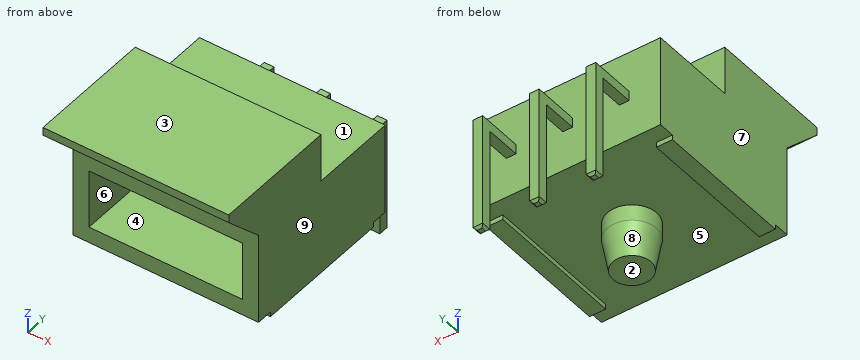
from build123d import *

# Parameters (mm, degrees)
F0_W           = 11.5
F0_H           = 10.66
F0_R           = 1.525
F1_DEPTH       = 5.65
F2_DEPTH       = 3
F3_SIZE2       = 0.3526539614
F3_SIZE        = 2
F4_W           = 9.5
F4_H           = 3.65
F5_DEPTH       = 7
F7_W           = 4.5
F7_H           = 0.6
F7_W_2         = 0.6
F7_H_2         = 4
F7_H_3         = 2.525
F7_W_3         = 5.86
F8_DEPTH       = 0.3
F8_DEPTH_BACK  = 0.3
F10_W          = 10.36
F10_H          = 0.6
F10_W_2        = 0.6
F10_H_2        = 6.525
F11_DEPTH      = 0.3
F11_DEPTH_BACK = 0.3
F13_W          = 10.36
F13_H          = 0.6
F13_W_2        = 0.6
F13_H_2        = 6.525
F14_DEPTH      = 0.3
F14_DEPTH_BACK = 0.3
F15_SIZE       = 0.15
F16_W          = 1
F16_H          = 8.66
F17_DEPTH      = 0.3
F19_DEPTH      = 11.5


with BuildPart() as f1:
    # F0 (on Top) → F1 (new body)
    with BuildSketch(Plane.XY):
        with Locations((0, -2.5)):
            Rectangle(F0_W, F0_H)
        with Locations((0, -2.58)):
            Circle(F0_R, mode=Mode.SUBTRACT)
        with Locations((0, -2.58)):
            Circle(F0_R)
    extrude(amount=F1_DEPTH)

    # F0 (on Top) → F2 (join)
    with BuildSketch(Plane.XY):
        with Locations((0, -2.58)):
            Circle(F0_R)
    extrude(amount=-F2_DEPTH)

    # F3
    f3_edges = [f1.edges().sort_by_distance(p)[0] for p in [
        (-1.525, -2.58, -3),
    ]]
    f3_side = f1.faces().sort_by_distance((-1.525, -2.58, -1.5))[0]
    chamfer(f3_edges, length=F3_SIZE, length2=F3_SIZE2, reference=f3_side)

    # F4 (on face) → F5 (cut)
    with BuildSketch(Plane.XZ.offset(7.83)):
        with Locations((0, 2.825)):
            Rectangle(F4_W, F4_H)
    extrude(amount=-F5_DEPTH, mode=Mode.SUBTRACT)

    # F7 (on mid) → F8 (join, two sides)
    with BuildSketch(Plane.YZ) as f8_sk:
        with Locations((-3.08, 2.825)):
            Rectangle(F7_W, F7_H)
        with Locations((5.33, 2.825)):
            Rectangle(F7_W_2, F7_H)
        with Locations((5.33, -2)):
            Rectangle(F7_W_2, F7_H_2)
        with Locations((5.33, 1.2625)):
            Rectangle(F7_W_2, F7_H_3)
        with Locations((2.1, 2.825)):
            Rectangle(F7_W_3, F7_H)
    extrude(amount=F8_DEPTH)
    extrude(f8_sk.sketch, amount=-F8_DEPTH_BACK)

    # F10 (on offset) → F11 (join, two sides)
    with BuildSketch(Plane.YZ.offset(3.5)) as f11_sk:
        with Locations((-0.15, 2.825)):
            Rectangle(F10_W, F10_H)
        with Locations((5.33, 2.825)):
            Rectangle(F10_W_2, F10_H)
        with Locations((5.33, -0.7375)):
            Rectangle(F10_W_2, F10_H_2)
    extrude(amount=F11_DEPTH)
    extrude(f11_sk.sketch, amount=-F11_DEPTH_BACK)

    # F13 (on offset) → F14 (join, two sides)
    with BuildSketch(Plane.YZ.offset(-3.5)) as f14_sk:
        with Locations((-0.15, 2.825)):
            Rectangle(F13_W, F13_H)
        with Locations((5.33, 2.825)):
            Rectangle(F13_W_2, F13_H)
        with Locations((5.33, -0.7375)):
            Rectangle(F13_W_2, F13_H_2)
    extrude(amount=F14_DEPTH)
    extrude(f14_sk.sketch, amount=-F14_DEPTH_BACK)

    # F15
    f15_edges = [f1.edges().sort_by_distance(p)[0] for p in [
        (-3.5, 5.03, -4),
        (-3.8, 5.33, -4),
        (-3.5, 5.63, -4),
        (-3.2, 5.33, -4),
        (-0.3, 5.33, -4),
        (0, 5.03, -4),
        (0.3, 5.33, -4),
        (0, 5.63, -4),
        (3.5, 5.03, -4),
        (3.2, 5.33, -4),
        (3.8, 5.33, -4),
        (3.5, 5.63, -4),
        (-3.2, -5.33, 2.825),
        (-3.5, -5.33, 3.125),
        (-3.8, -5.33, 2.825),
        (-3.5, -5.33, 2.525),
        (0, -5.33, 3.125),
        (-0.3, -5.33, 2.825),
        (0.3, -5.33, 2.825),
        (0, -5.33, 2.525),
        (3.2, -5.33, 2.825),
        (3.5, -5.33, 3.125),
        (3.8, -5.33, 2.825),
        (3.5, -5.33, 2.525),
    ]]
    chamfer(f15_edges, length=F15_SIZE)

    # F16 (on face) → F17 (join)
    with BuildSketch(Plane(origin=(0, 0, 0), x_dir=(1, 0, 0), z_dir=(0, 0, -1))):
        with Locations((5.25, 2.5)):
            Rectangle(F16_W, F16_H)
        with Locations((-5.25, 2.5)):
            Rectangle(F16_W, F16_H)
    extrude(amount=F17_DEPTH)

    # F18 (on face) → F19 (join, through all)
    with BuildSketch(Plane.YZ.offset(5.75)):
        Polygon((-10.34, 8.16), (-7.83, 5.65), (-2.58, 5.65), (-2.58, 8.66), (-10.34, 8.66), align=None)
    extrude(amount=-F19_DEPTH)


solid = f1.part
Could you check a few things on this model? Use its own coordinates, in mm. Face numbers are marked on the shaded views. A direction names the side the tool comes from. Give positions to 0.01 mm unless a question says otherwise; leave off trailing zeros. Order: outer loops, then holes, each group sorted by start corner. A loop starts at its lowest first (then second) coordinate and runs counter-clockwise, first axis right, second up.
1. For the marked faces 1, 2, 3, 4 and 5, which set-ups out of +Z, -Z, +X, -X, +Y, -Y let a thin tool reach every point of the face, with its end or its side?
2. Suppose I cut it at B-B (y = -6). List the corners of the cut face in (x, z) for me.
3. I need wall thicknesses on L1, parallel to Z at x = 0, y = -4.5 (3 decimals); L2, parallel to X at y = -2.25, z = 4.5; L3, parallel to Z at x = 4, y = -2. Which ranges of each line are inside material? Lowest first, please.
4. Suppose I cut it at C-C (z = 4). List the corners of the cut face in (x, y) for me.
5. Suppose I cut it at A-A (z = -0.75). List the corners of the cut face in (x, y) for me (3 decimals).
6. Suppose I cut it at D-D (x = -2). List the corners of the cut face in (y, z) for me.
7. Will these pins go through, and if not, where does the flat tip stop? P1, Ø5, axis at x = -3, y = -1, coming from the +Z side; P2, Ø0.7, axis at x = 3.5, y = 4, coming from the +Z side (3 decimals); P3, Ø2, axis at y = 5, z = -0.5, coming from the -X side.
8. We'd pull the mould along X, two halves only. Please class the marked faces 6, 7, 8 and 9: pulls with the +X half, pulls with the -X half, needs draft (parallel to the pull), parting line crosses it, or undercut.
Solved:
1. face 1: +Z, +X, -X, +Y
1. face 2: -Z, +X, -X, -Y
1. face 3: +Z, +X, -X, +Y, -Y
1. face 4: -Y
1. face 5: -Z
2. outline: (-5.75, -0.3) - (-4.75, -0.3) - (-4.75, 0) - (4.75, 0) - (4.75, -0.3) - (5.75, -0.3) - (5.75, 8.66) - (-5.75, 8.66) - close; hole (-4.75, 1) - (4.75, 1) - (4.75, 4.65) - (-4.75, 4.65) - close
3. L1: z = 0 to 1, 2.525 to 3.125, 4.65 to 8.66
3. L2: x = -5.75 to -4.75, 4.75 to 5.75
3. L3: z = 0 to 1, 4.65 to 5.65
4. outline: (-5.75, -7.83) - (-4.75, -7.83) - (-4.75, -0.83) - (4.75, -0.83) - (4.75, -7.83) - (5.75, -7.83) - (5.75, 2.83) - (-5.75, 2.83) - close
5. outline: (-3.8, 5.03) - (-3.2, 5.03) - (-3.2, 5.63) - (-3.8, 5.63) - close; circle Ø3.05 at (0, -2.58); (-0.3, 5.03) - (0.3, 5.03) - (0.3, 5.63) - (-0.3, 5.63) - close; (3.2, 5.03) - (3.8, 5.03) - (3.8, 5.63) - (3.2, 5.63) - close
6. outline: (-10.34, 8.16) - (-7.83, 5.65) - (-7.83, 4.65) - (-0.83, 4.65) - (-0.83, 1) - (-7.83, 1) - (-7.83, 0) - (2.83, 0) - (2.83, 5.65) - (-2.58, 5.65) - (-2.58, 8.66) - (-10.34, 8.66) - close
7. P1: stops at z = 8.66
7. P2: stops at z = 3.125
7. P3: stops at x = -3.8
8. face 6: undercut
8. face 7: pulls with the -X half
8. face 8: parting line crosses it
8. face 9: pulls with the +X half
